```python
from build123d import *

# Parameters (mm, degrees)
F1_DEPTH = 100
F2_SIZE2 = 15
F2_SIZE  = 15
F3_W     = 8.609191
F3_H     = 79.327516
F3_W_2   = 51.655116
F4_DEPTH = 17.001
F5_W     = 26.5
F5_H     = 2.5
F6_DEPTH = 2


with BuildPart() as f1:
    # F0 (on Front) → F1 (new body)
    with BuildSketch(Plane.XZ):
        Polygon((7, 0), (0, 0), (0, -17), (208, -17), (208, 0), (201, 0), (201, -11), (191.25, -11), (191.25, 0), (184.25, 0), (184.25, -11), (174.5, -11), (174.5, 0), (167.5, 0), (167.5, -11), (157.75, -11), (157.75, 0), (150.75, 0), (150.75, -11), (141, -11), (141, 0), (134, 0), (134, -11), (124.25, -11), (124.25, 0), (117.25, 0), (117.25, -11), (107.5, -11), (107.5, 0), (100.5, 0), (100.5, -11), (90.75, -11), (90.75, 0), (83.75, 0), (83.75, -11), (74, -11), (74, 0), (67, 0), (67, -11), (57.25, -11), (57.25, 0), (50.25, 0), (50.25, -11), (40.5, -11), (40.5, 0), (33.5, 0), (33.5, -11), (23.75, -11), (23.75, 0), (16.75, 0), (16.75, -11), (7, -11), align=None)
    extrude(amount=F1_DEPTH)

    # F2
    f2_edges = [f1.edges().sort_by_distance(p)[0] for p in [
        (0, 0, -8.5),
    ]]
    chamfer(f2_edges, length=F2_SIZE, length2=F2_SIZE2)

    # F3 (on Top) → F4 (cut, through all)
    with BuildSketch(Plane.XY):
        Polygon((214.614749, -116.838969), (214.614749, 11.068958), (41.201111, 11.068958), (41.201111, -37.511453), (49.810302, -37.511453), (49.810302, -116.838969), align=None)
        with Locations((45.505707, -77.175211)):
            Rectangle(F3_W, F3_H)
        with Locations((15.373553, -77.175211)):
            Rectangle(F3_W_2, F3_H)
    extrude(amount=-F4_DEPTH, mode=Mode.SUBTRACT)

    # F5 (on face) → F6 (join)
    with BuildSketch(Plane.XZ.offset(37.511453)):
        with Locations((20.25, -9.75)):
            Rectangle(F5_W, F5_H)
    extrude(amount=-F6_DEPTH)


solid = f1.part
```
The listing builds one solid part. Answer for the finished solid, in the listing's coordinates (mm). A direction names the side the tool comes from. Coordinates: 2 decimals unless noted, no trailing zeros. Loops run counter-clockwise (first coordinate to the right, second up) from the corner with the lowest first, then second, coordinate; pieces in that order, holes last. Notation, with made-up numbers: M -17.5,-35 L 21.5,-35 A20 cw 21.5,-14 Z; hole C 53.5,-35.5 d5. An arc over 180 degrees is marked long. Answer as CSV lines item,"result". Start each with the question number.
(1) For faces 1 (the flat face through (12, -37, -8.5)), 2 (the flat face through (12, -35.511, -10)), 3 (the flat face through (41.201, -18, -14)), determine the directions among +Z, -Z, +X, -X, +Y, -Y from which every point of the face is accessible in a straight line to the end or side of a thin tool.
(2) The part is cut by section B-B (y = -12). Give the vertices of the cut face in (x, z), and give its area (3 significant figures).
(3) The part is cut by section A-A (z = -5.75). Give the vertices of the cut face in (x, y).
(4) Given pin 1 (9 mm diameter, centred on y = -27.5, z = -3, fed in from +X); pin 2 (8 mm diameter, centred on x = 27.5, y = -20, fed in from +Z); pin 3 (1.6 mm diameter, centred on x = 13, y = -36.5, fed in from +Z); pin 4 (1 mm diameter, centred on x = 27, y = -8.5, fed in from +Z), each flat-ended and moving along its own axis, determine where each tip first touches the part or whether it passes through.
(5) Find the intervals of material crossed by L1, parallel to X at y = -25, z = -1.25; L2, parallel to Z at x = 9, y = -25.5; L3, parallel to X at y = -5, z = -12.5, in increasing order. Write a range as [from, to].
(6) The part is cut by section C-C (x = 14). Give the vertices of the cut face in (y, z), and give its area (3 significant figures).
(7) The mould has two halves that part along X. Classify faces 4 (the flat face through (6, -9, -10)), 5 (the flat face through (20, -37.511, -10)), 6 (the flat face through (29, -35.511, -10)), 7 (the flat face through (40.5, -18, -6)): pulls with the +X half, pulls with the -X half, needs draft (parallel to the pull), parting line crosses it, or undercut.
(8) The part is cut by section D-D (z = -13). Give the vertices of the cut face in (x, y).
Determined:
1,face 1,"+Z, +Y, -Y"
1,face 2,"+Z, +Y"
1,face 3,"+Z, -Z, +X, +Y, -Y"
2,outline,"M 3,-17 L 41.2,-17 L 41.2,-11 L 40.5,-11 L 40.5,0 L 33.5,0 L 33.5,-11 L 23.75,-11 L 23.75,0 L 16.75,0 L 16.75,-11 L 7,-11 L 7,0 L 3,0 Z"
2,area,"427 mm2"
3,outline,"M 0,-37.51 L 7,-37.51 L 7,-8 L 0,-15 Z; M 16.75,-37.51 L 23.75,-37.51 L 23.75,0 L 16.75,0 Z; M 33.5,-37.51 L 40.5,-37.51 L 40.5,0 L 33.5,0 Z"
4,pin 1,"x = 40.5"
4,pin 2,"z = 0"
4,pin 3,"z = -8.5"
4,pin 4,"z = -11"
5,L1,"[0, 7], [16.75, 23.75], [33.5, 40.5]"
5,L2,"[-17, -11]"
5,L3,"[10, 41.2]"
6,outline,"M -37.51,-17 L -1,-17 L -1,-11 L -35.51,-11 L -35.51,-8.5 L -37.51,-8.5 Z"
6,area,"224 mm2"
7,face 4,"pulls with the -X half"
7,face 5,"needs draft"
7,face 6,"undercut"
7,face 7,"pulls with the +X half"
8,outline,"M 0,-37.51 L 41.2,-37.51 L 41.2,0 L 15,0 L 0,-15 Z"
